```python
from build123d import *

# Parameters (mm, degrees)
SKETCH1_R           = 13
BOSS_EXTRUDE1_DEPTH = 2.8
SKETCH2_R           = 13
SKETCH2_R_2         = 3
BOSS_EXTRUDE2_DEPTH = 2.5
CHAMFER1_SIZE       = 1
FILLET1_R           = 0.25


with BuildPart() as part:
    # Sketch1 → Boss-Extrude1 (new body)
    with BuildSketch(Plane(origin=(0, 0, 0), x_dir=(1, 0, 0), z_dir=(0, 1, 0))):
        Circle(SKETCH1_R)
        Polygon((0, -9.959292144), (8.625, -4.979646072), (8.625, 4.979646072), (0, 9.959292144), (-8.625, 4.979646072), (-8.625, -4.979646072), align=None, mode=Mode.SUBTRACT)
    extrude(amount=BOSS_EXTRUDE1_DEPTH)

    # Sketch2 → Boss-Extrude2 (add)
    with BuildSketch(Plane(origin=(0, 2.8, 0), x_dir=(1, 0, 0), z_dir=(0, 1, 0))):
        Circle(SKETCH2_R)
        Circle(SKETCH2_R_2, mode=Mode.SUBTRACT)
    extrude(amount=BOSS_EXTRUDE2_DEPTH)

    # Chamfer1
    chamfer1_edges = [part.edges().sort_by_distance(p)[0] for p in [
        (-13, 5.3, 0),
    ]]
    chamfer(chamfer1_edges, length=CHAMFER1_SIZE)

    # Fillet1
    fillet1_edges = [part.edges().sort_by_distance(p)[0] for p in [
        (-3, 2.8, 0),
    ]]
    fillet(fillet1_edges, radius=FILLET1_R)


solid = part.part
```
Verification items for the finished model (mm, model axes). A direction names the side the tool comes from. Coordinates: 2 decimals unless noted, no trailing zeros. Loops run counter-clockwise (first coordinate to the right, second up) from the corner with the lowest first, then second, coordinate; pieces in that order, holes last. Notation, with made-up numbers: (49, 88) - (73, 88) arc R11 ccw to (73, 107) - close; hole circle Ø4 at (18.5, 60). An arc over 180 degrees is marked (long way). Return JSON: item names as keys, results as strings.
1. Tool access check on faces 4 (the flat face through (0, 2.8, 4)), 5 (the flat face through (2.5, 5.3, 2.5)). Record the directions out of +Z, -Z, +X, -X, +Y, -Y that give a thin tool (end or side, any length) a straight path to the whole face; none if there is none.
Established:
{"face 4": "-Y", "face 5": "+Z, -Z, +X, -X, +Y"}
2. Go/stop test with flat-tipped pins: pin 1 (0.8 mm diameter, centred on y = 1.5, z = 2, fed in from +X); pin 2 (5.5 mm diameter, centred on x = 0, z = 0, fed in from -Y); pin 3 (3 mm diameter, centred on y = 2, z = 5, fed in from -X); pin 4 (1.5 mm diameter, centred on x = 5, y = 4.5, fed in from -Z). Record where each tip stops, or that it passes through.
Established:
{"pin 1": "stops at x = 12.9", "pin 2": "passes through", "pin 3": "stops at x = -12.52", "pin 4": "stops at z = -12.28"}
3. Thickness scan on L1, parallel to X at y = 3.6, z = 0; L2, parallel to Y at x = 1.25, z = 5.75. Record the ranges inside material, lowest first.
Established:
{"L1": "x = -13 to -3, 3 to 13", "L2": "y = 2.8 to 5.3"}
4. Section check A-A, the plane z = 0. Record the boundary of the cut face in (x, y) (3 decimals), then the cut area to 3 significant figures.
Established:
{"outline": "(-13, 0) - (-8.625, 0) - (-8.625, 2.8) - (-3.25, 2.8) arc R0.25 ccw to (-3, 3.05) - (-3, 5.3) - (-12, 5.3) - (-13, 4.3) - close; (3, 3.05) arc R0.25 ccw to (3.25, 2.8) - (8.625, 2.8) - (8.625, 0) - (13, 0) - (13, 4.3) - (12, 5.3) - (3, 5.3) - close", "area": "73.5 mm2"}
5. Section check B-B, the plane y = 0.45. Record the boundary of the cut face in (x, z) (3 decimals), then the cut area to 3 significant figures.
Established:
{"outline": "circle Ø26 at (0, 0); hole (-8.625, -4.98) - (0, -9.959) - (8.625, -4.98) - (8.625, 4.98) - (0, 9.959) - (-8.625, 4.98) - close", "area": "273 mm2"}
6. Mould release check, pull along X, two halves, no side actions. Record for faces 1 (the flat face through (-3.1, 0, 8.5)), 2 (the flat face through (4.373, 1.38, -7.435)), 3 (the cylindrical face through (-10.316, 2.12, 7.91)): +X half, -X half, draft (parallel to the pull), parting line (faces both ways), or undercut.
Established:
{"face 1": "draft", "face 2": "undercut", "face 3": "parting line"}
